Can you work these out from the model? Positions are in its coordinate system, mm. Give positions to 0.01 mm unless a question says otherwise; leave off trailing zeros. Loops run counter-clockwise (first coordinate to the right, second up) from the corner with the lowest first, then second, coordinate; pieces in that order, holes last. Notation, with made-up numbers: (52.5, -29.75) - (76.5, -29.75) arc R19 cw to (76.5, -14.75) - close; hole circle Ø9 at (-24, 65.25). An arc over 180 degrees is marked (long way). Use a Markdown table: item, result. Add a question column.
```python
from build123d import *

# Parameters (mm, degrees)
F0_W     = 553
F0_H     = 452
F0_W_2   = 457
F0_H_2   = 354
F1_DEPTH = 22.5
F2_SIZE2 = 13
F2_SIZE  = 6
F3_SIZE2 = 7
F3_SIZE  = 17


with BuildPart() as f1:
    # F0 (on Front) → F1 (new body, symmetric)
    with BuildSketch(Plane.XZ):
        Rectangle(F0_W, F0_H)
        Rectangle(F0_W_2, F0_H_2, mode=Mode.SUBTRACT)
    extrude(amount=F1_DEPTH, both=True)

    # F2
    f2_edges = [f1.edges().sort_by_distance(p)[0] for p in [
        (0, -22.5, -177),
        (-228.5, -22.5, 0),
        (228.5, -22.5, 0),
        (0, -22.5, 177),
    ]]
    chamfer(f2_edges, length=F2_SIZE, length2=F2_SIZE2)

    # F3
    f3_edges = [f1.edges().sort_by_distance(p)[0] for p in [
        (0, 22.5, -177),
        (-228.5, 22.5, 0),
        (0, 22.5, 177),
        (228.5, 22.5, 0),
    ]]
    chamfer(f3_edges, length=F3_SIZE, length2=F3_SIZE2)


solid = f1.part
```
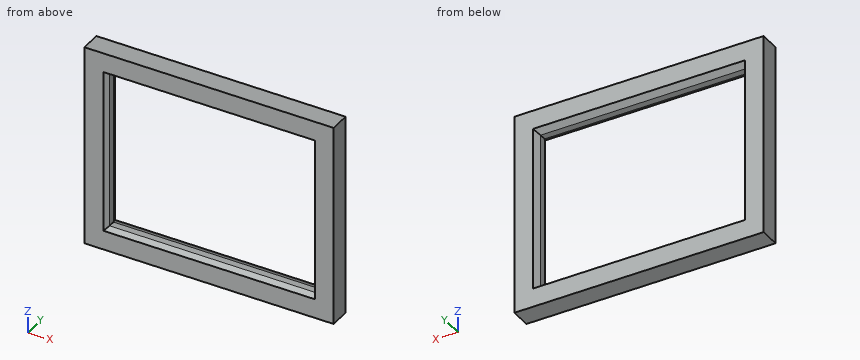
1. Suppose I cut it at B-B (z = -35.5). List the corners of the cut face in (x, y) for me, and give its area (3 significant figures).
2. Please list where these lines run through material, in increasing order: line 1 along Z through (x, y) = (180.5, 0.5); line 2 along X through (y, z) = (-8.5, -63); line 3 along X through (y, z) = (20, 96). Write a range as [from, to].
3. Suppose I cut it at A-A (y = -0.5). List the corners of the cut face in (x, z) for me.
4. Suppose I cut it at C-C (x = 208). List the corners of the cut face in (y, z) for me.
Results below:
| question | item | result |
|---|---|---|
| 1 | outline | (-276.5, -22.5) - (-234.5, -22.5) - (-228.5, -9.5) - (-228.5, 5.5) - (-235.5, 22.5) - (-276.5, 22.5) - close; (228.5, -9.5) - (234.5, -22.5) - (276.5, -22.5) - (276.5, 22.5) - (235.5, 22.5) - (228.5, 5.5) - close |
| 1 | area | 4,120 mm² |
| 2 | line 1 | [-226, -177], [177, 226] |
| 2 | line 2 | [-276.5, -228.5], [228.5, 276.5] |
| 2 | line 3 | [-276.5, -234.47], [234.47, 276.5] |
| 3 | outline | (-276.5, -226) - (276.5, -226) - (276.5, 226) - (-276.5, 226) - close; hole (-228.5, -177) - (228.5, -177) - (228.5, 177) - (-228.5, 177) - close |
| 4 | outline | (-22.5, -226) - (22.5, -226) - (22.5, -184) - (5.5, -177) - (-9.5, -177) - (-22.5, -183) - close; (-22.5, 183) - (-9.5, 177) - (5.5, 177) - (22.5, 184) - (22.5, 226) - (-22.5, 226) - close |
